from build123d import *
from build123d.topology import SkipClean

# Parameters (mm, degrees)
SKETCH1_R           = 22
BOSS_EXTRUDE1_DEPTH = 1
SKETCH2_R           = 20
CUT_EXTRUDE1_DEPTH  = 1
SKETCH3_R           = 20
BOSS_EXTRUDE2_DEPTH = 1
BOSS_EXTRUDE3_REACH = 52.675
SKETCH5_R           = 20
SKETCH5_R_2         = 19.004147065
BOSS_EXTRUDE4_DEPTH = 10
CUT_EXTRUDE2_DEPTH  = 10


with BuildPart() as part:
    # Sketch1 → Boss-Extrude1 (new body)
    with BuildSketch(Plane(origin=(0, 0, 0), x_dir=(1, 0, 0), z_dir=(0, 1, 0))):
        with Locations(Location((0, 0, 0), (0, 0, 270))):
            Circle(SKETCH1_R)
    extrude(amount=BOSS_EXTRUDE1_DEPTH)

    # Sketch2 → Cut-Extrude1 (cut)
    with BuildSketch(Plane(origin=(0, 1, 0), x_dir=(1, 0, 0), z_dir=(0, 1, 0))):
        with Locations(Location((0, 0, 0), (0, 0, 270))):
            Circle(SKETCH2_R)
    extrude(amount=-CUT_EXTRUDE1_DEPTH, mode=Mode.SUBTRACT)

    # Boss-Extrude3: up to this face of the body (flat: up to its plane)
    boss_extrude3_end = Plane(part.part.faces().sort_by_distance((0, 1, -21.377746033))[0])
    # Sketch4 → Boss-Extrude3 (add, up to the picked face)
    with BuildSketch(Plane(origin=(0, -39, 0), x_dir=(1, 0, 0), z_dir=(0, 1, 0)), mode=Mode.PRIVATE) as boss_extrude3_sk1:
        with BuildLine():
            Line((-5.176380902, 19.318516526), (-4.834360759, 18.378823905))
            ThreePointArc((-4.834360759, 18.378823905), (-2.437308738, 18.847061792), (0, 19.004005159))
            ThreePointArc((0, 19.004005159), (2.437764249, 18.84700288), (4.835249142, 18.378590202))
            Line((4.835249142, 18.378590202), (5.176380902, 19.318516526))
            ThreePointArc((5.176380902, 19.318516526), (2.610523844, 19.828897227), (0, 20))
            ThreePointArc((0, 20), (-2.610523844, 19.828897227), (-5.176380902, 19.318516526))
        make_face()
    boss_extrude3_tool1 = split(extrude(boss_extrude3_sk1.sketch, amount=BOSS_EXTRUDE3_REACH, mode=Mode.PRIVATE), bisect_by=boss_extrude3_end, keep=Keep.BOTH, mode=Mode.PRIVATE)
    # Sketch4 → Boss-Extrude3 (add, up to the picked face)
    with BuildSketch(Plane(origin=(0, -39, 0), x_dir=(1, 0, 0), z_dir=(0, 1, 0)), mode=Mode.PRIVATE) as boss_extrude3_sk2:
        with BuildLine():
            Line((19.318516526, 5.176380902), (18.378823905, 4.834360759))
            ThreePointArc((18.378823905, 4.834360759), (18.847061792, 2.437308738), (19.004005159, 0))
            ThreePointArc((19.004005159, 0), (18.84700288, -2.437764249), (18.378590202, -4.835249142))
            Line((18.378590202, -4.835249142), (19.318516526, -5.176380902))
            ThreePointArc((19.318516526, -5.176380902), (19.828897227, -2.610523844), (20, 0))
            ThreePointArc((20, 0), (19.828897227, 2.610523844), (19.318516526, 5.176380902))
        make_face()
    boss_extrude3_tool2 = split(extrude(boss_extrude3_sk2.sketch, amount=BOSS_EXTRUDE3_REACH, mode=Mode.PRIVATE), bisect_by=boss_extrude3_end, keep=Keep.BOTH, mode=Mode.PRIVATE)
    # Sketch4 → Boss-Extrude3 (add, up to the picked face)
    with BuildSketch(Plane(origin=(0, -39, 0), x_dir=(1, 0, 0), z_dir=(0, 1, 0)), mode=Mode.PRIVATE) as boss_extrude3_sk3:
        with BuildLine():
            Line((5.176380902, -19.318516526), (4.834360759, -18.378823905))
            ThreePointArc((4.834360759, -18.378823905), (2.437308738, -18.847061792), (0, -19.004005159))
            ThreePointArc((0, -19.004005159), (-2.437764249, -18.84700288), (-4.835249142, -18.378590202))
            Line((-4.835249142, -18.378590202), (-5.176380902, -19.318516526))
            ThreePointArc((-5.176380902, -19.318516526), (-2.610523844, -19.828897227), (0, -20))
            ThreePointArc((0, -20), (2.610523844, -19.828897227), (5.176380902, -19.318516526))
        make_face()
    boss_extrude3_tool3 = split(extrude(boss_extrude3_sk3.sketch, amount=BOSS_EXTRUDE3_REACH, mode=Mode.PRIVATE), bisect_by=boss_extrude3_end, keep=Keep.BOTH, mode=Mode.PRIVATE)
    # Sketch4 → Boss-Extrude3 (add, up to the picked face)
    with BuildSketch(Plane(origin=(0, -39, 0), x_dir=(1, 0, 0), z_dir=(0, 1, 0)), mode=Mode.PRIVATE) as boss_extrude3_sk4:
        with BuildLine():
            Line((-19.318516526, -5.176380902), (-18.378823905, -4.834360759))
            ThreePointArc((-18.378823905, -4.834360759), (-18.847061792, -2.437308738), (-19.004005159, 0))
            ThreePointArc((-19.004005159, 0), (-18.84700288, 2.437764249), (-18.378590202, 4.835249142))
            Line((-18.378590202, 4.835249142), (-19.318516526, 5.176380902))
            ThreePointArc((-19.318516526, 5.176380902), (-19.828897227, 2.610523844), (-20, 0))
            ThreePointArc((-20, 0), (-19.828897227, -2.610523844), (-19.318516526, -5.176380902))
        make_face()
    boss_extrude3_tool4 = split(extrude(boss_extrude3_sk4.sketch, amount=BOSS_EXTRUDE3_REACH, mode=Mode.PRIVATE), bisect_by=boss_extrude3_end, keep=Keep.BOTH, mode=Mode.PRIVATE)


with BuildPart() as body_2:
    # Sketch3 → Boss-Extrude2 (new body)
    with BuildSketch(Plane(origin=(0, -40, 0), x_dir=(1, 0, 0), z_dir=(0, 1, 0))):
        with Locations(Location((0, 0, 0), (0, 0, 270))):
            Circle(SKETCH3_R)
    extrude(amount=BOSS_EXTRUDE2_DEPTH)


with BuildPart() as part_1:
    add(part.part)

    add(body_2.part)  # Boss-Extrude3 merges body 2
    add(boss_extrude3_tool1.solids().sort_by(Axis((0.000224, -39, -19.289315), (0, 1, 0)))[0])
    add(boss_extrude3_tool2.solids().sort_by(Axis((19.289315, -39, 0.000224), (0, 1, 0)))[0])
    add(boss_extrude3_tool3.solids().sort_by(Axis((-0.000224, -39, 19.289315), (0, 1, 0)))[0])
    add(boss_extrude3_tool4.solids().sort_by(Axis((-19.289315, -39, -0.000224), (0, 1, 0)))[0])

    # Sketch5 → Boss-Extrude4 (add)
    with SkipClean():  # the faces are left unmerged after this step: merging them gives an invalid solid
        with BuildSketch(Plane(origin=(0, -39, 0), x_dir=(1, 0, 0), z_dir=(0, 1, 0))):
            with Locations(Location((0, 0, 0), (0, 0, 105))):
                Circle(SKETCH5_R)
            Circle(SKETCH5_R_2, mode=Mode.SUBTRACT)
        extrude(amount=BOSS_EXTRUDE4_DEPTH)

    # Sketch6 → Cut-Extrude2 (cut)
    with SkipClean():  # the faces are left unmerged after this step: merging them gives an invalid solid
        with BuildSketch(Plane.XZ.offset(40)):
            with BuildLine():
                ThreePointArc((-18, 5), (0, 18.681541692), (18, 5))
                Line((18, 5), (-18, 5))
            make_face()
            with BuildLine():
                Line((-18, -5), (18, -5))
                ThreePointArc((18, -5), (0, -18.681541692), (-18, -5))
            make_face()
        extrude(amount=-CUT_EXTRUDE2_DEPTH, mode=Mode.SUBTRACT)


solid = part_1.part
The model under review builds one solid part; all positions refer to its coordinate system, in mm. A direction names the side the tool comes from. Round coordinates to 2 decimals unless told otherwise and drop trailing zeros. Loops run counter-clockwise (first coordinate to the right, second up) from the corner with the lowest first, then second, coordinate; pieces in that order, holes last. Notation, with made-up numbers: (28, -2) -> (32, -2) arc R26 ccw to (32, 31) -> close; hole circle Ø4 at (83, 46). An arc over 180 degrees is marked (long way). Answer as CSV lines item,"result".
1) To check wall thickness, follow line 1 along Z through (x, y) = (0.5, -14.5); line 2 along Z through (x, y) = (-13, -29.5); line 3 along X through (y, z) = (-26, -3.5). State the ranges of each line that lie inside material, in increasing order. Write a range as from..to.
Geometry results:
line 1,"z = -19.99..-19, 19..19.99"
line 2,"z = -15.2..-13.86, 13.86..15.2"
line 3,"x = -19.69..-18.68, 18.68..19.69"
2) Add section A-A on y = -1.5. Write out the cut boundary in (x, z), plus the area to 3 significant figures.
Geometry results:
outline,"(-19.32, -5.18) -> (-18.38, -4.84) arc R19 cw to (-18.38, 4.83) -> (-19.32, 5.18) arc R20 ccw to start; (-5.18, -19.32) arc R20 ccw to (5.18, -19.32) -> (4.84, -18.38) arc R19 cw to (-4.83, -18.38) -> close; (-5.18, 19.32) -> (-4.84, 18.38) arc R19 cw to (4.83, 18.38) -> (5.18, 19.32) arc R20 ccw to start; (18.38, -4.83) -> (19.32, -5.18) arc R20 ccw to (19.32, 5.18) -> (18.38, 4.84) arc R19 cw to start"
area,"40.3 mm²"
3) For P1, Ø10, axis at y = -31, z = 17, coming from the +X side; P2, Ø4.5, axis at x = -13, z = 11.5, coming from the +Y side; P3, Ø6, axis at y = -31.5, z = -13.5, coming from the +X side, all flat-tipped, find the tip position at first contact; note any pin that passes through.
Geometry results:
P1,"stops at x = 16"
P2,"stops at y = -29"
P3,"stops at x = 17.02"
4) Draft analysis for pull direction X (two halves, no side actions). For faces 4 (the face through (20, 1, 2)), 5 (the face through (-13.537, -34.07, 13.338)), 6 (the face through (-21.477, 0.493, -4.769)), state which applies: pulls with the +X half, pulls with the -X half, needs draft (parallel to the pull), parting line crosses it, or undercut.
Geometry results:
face 4,"needs draft"
face 5,"undercut"
face 6,"parting line crosses it"
5) Tool access review of faces 1 (the face through (-18, 0, 10)), 2 (the face through (0, -40, 0)), 3 (the face through (-14.245, 0.507, 14.038)): name each direction out of +Z, -Z, +X, -X, +Y, -Y from which nothing blocks a thin tool from reaching the whole face with its end or side.
Geometry results:
face 1,"-Y"
face 2,"+Z, -Z, +X, -X, -Y"
face 3,"+Y"
